Could you check a few things on this model? Use its own coordinates, in mm. A direction names the side the tool comes from. Coordinates: 2 decimals unless noted, no trailing zeros. Order: outer loops, then holes, each group sorted by start corner. A loop starts at its lowest first (then second) coordinate and runs counter-clockwise, first axis right, second up. Notation, with made-up numbers: (44, -19.5) -> (77, -19.5) arc R18 cw to (77, 13.5) -> close; hole circle Ø11 at (46, 6.25). An arc over 180 degrees is marked (long way). Use a Markdown table: item, result. Add a question column.
1) Will these pins go through, and if not, where does the flat tip stop? pin 1 Ø3 at (x, y) = (37, -4.5) entering from +Z; pin 2 Ø4 at (x, y) = (50.8, 0) entering from -Z.
2) If we section it at C-C (y = 0): Give the number of separate pieces and of enclosed holes in the cut face, plus the area to 3 significant figures.
3) Thinking about a two-plate mould opening in Y: for faces 1 (the flat face through (-2, -3, 2.476)), 2 (the cylindrical face through (56.515, -0.087, 0.017)), 3 (the cylindrical face through (23.1, -0.95, 0.62)), which applies, +Y half, -Y half, draft (parallel to the pull), parting line (faces both ways), or undercut?
4) Which directions (+Z, -Z, +X, -X, +Y, -Y) give clear straight access to the entire face, cutting with the end or side of a thin tool? Please do faces 4 (the flat face through (26, 5.588, 0)), 5 (the cylindrical face through (54.57, 0.17, 1.85)).
5) If we section it at A-A (x = 0): Write out the boundary of the cut face in (y, z) (1 decimal), plus the area to 3 significant figures.
6) If we section it at B-B (z = 0): Write out the boundary of the cut face in (x, y).
7) If I drill on L1, parallel to X at y = 0, z = 0.5 (3 decimals); L2, parallel to X at y = 0.5, z = 2.1; L3, parallel to X at y = -1, z = 2.2, over which ranges is the centre line in solid material (lowest first)? Write a range as [from, to].
```python
from build123d import *

# Parameters (mm, degrees)
BOSS_EXTRUDE1_DEPTH = 2.413
SKETCH2_W           = 3.7719
SKETCH2_H           = 1.27
SKETCH3_W           = 3.7719
SKETCH3_H           = 1.27
SKETCH4_W           = 3.7719
SKETCH4_H           = 1.27
HOLE1_D             = 4.97586
HOLE1_CSINK_D       = 6.35
HOLE1_CSINK_ANGLE   = 90
CHAMFER1_SIZE       = 0.68707


with BuildPart() as part:
    # Sketch1 → Boss-Extrude1 (new body)
    with BuildSketch(Plane.XY.offset(1.2065)):
        with BuildLine():
            Line((54.209515887, 5.588), (-3.409515887, 5.588))
            ThreePointArc((-3.409515887, 5.588), (-5.715, 0), (-3.409515887, -5.588))
            Line((-3.409515887, -5.588), (54.209515887, -5.588))
            ThreePointArc((54.209515887, -5.588), (56.515, 0), (54.209515887, 5.588))
        make_face()
    extrude(amount=-BOSS_EXTRUDE1_DEPTH)

    # Sketch2 → Revolve1 (revolve)
    with BuildSketch(Plane.XZ, mode=Mode.PRIVATE) as revolve1_sk:
        with Locations((27.28595, 1.8415)):
            Rectangle(SKETCH2_W, SKETCH2_H)
    revolve(revolve1_sk.sketch.rotate(Axis((25.4, 0, 2.4765), (0, 0, -1)), 180), axis=Axis((25.4, 0, 2.4765), (0, 0, -1)))

    # Sketch3 → Revolve2 (revolve)
    with BuildSketch(Plane.XZ, mode=Mode.PRIVATE) as revolve2_sk:
        with Locations((1.88595, 1.8415)):
            Rectangle(SKETCH3_W, SKETCH3_H)
    revolve(revolve2_sk.sketch.rotate(Axis((0, 0, 2.4765), (0, 0, -1)), 180), axis=Axis((0, 0, 2.4765), (0, 0, -1)))

    # Sketch4 → Revolve3 (revolve)
    with BuildSketch(Plane.XZ, mode=Mode.PRIVATE) as revolve3_sk:
        with Locations((52.68595, 1.8415)):
            Rectangle(SKETCH4_W, SKETCH4_H)
    revolve(revolve3_sk.sketch.rotate(Axis((50.8, 0, 2.4765), (0, 0, -1)), 180), axis=Axis((50.8, 0, 2.4765), (0, 0, -1)))

    # Hole1 (through all)
    with Locations(Plane.XY.offset(2.4765)):
        with Locations((0, 0), (25.4, 0), (50.8, 0)):
            CounterSinkHole(HOLE1_D / 2, HOLE1_CSINK_D / 2, counter_sink_angle=HOLE1_CSINK_ANGLE)

    # Chamfer1
    chamfer1_edges = [part.edges().sort_by_distance(p)[0] for p in [
        (53.28793, 0, -1.2065),
        (27.88793, 0, -1.2065),
        (2.48793, 0, -1.2065),
    ]]
    chamfer(chamfer1_edges, length=CHAMFER1_SIZE)


solid = part.part
```
Answer sheet:
| question | item | result |
|---|---|---|
| 1 | pin 1 | z = 1.21 |
| 1 | pin 2 | through |
| 2 | separate pieces | 4 |
| 2 | enclosed holes | 0 |
| 2 | area | 121 mm2 |
| 3 | face 1 | draft |
| 3 | face 2 | parting line |
| 3 | face 3 | undercut |
| 4 | face 4 | +Z, -Z, +X, -X, +Y |
| 4 | face 5 | +Z |
| 5 | outline | (-5.6, -1.2) -> (-3.2, -1.2) -> (-2.5, -0.5) -> (-2.5, 1.8) -> (-3.2, 2.5) -> (-3.8, 2.5) -> (-3.8, 1.2) -> (-5.6, 1.2) -> close; (2.5, -0.5) -> (3.2, -1.2) -> (5.6, -1.2) -> (5.6, 1.2) -> (3.8, 1.2) -> (3.8, 2.5) -> (3.2, 2.5) -> (2.5, 1.8) -> close |
| 5 | area | 17.3 mm2 |
| 6 | outline | (-3.41, -5.59) -> (54.21, -5.59) arc R7.92 ccw to (54.21, 5.59) -> (-3.41, 5.59) arc R7.92 ccw to start; hole circle Ø4.98 at (0, 0); hole circle Ø4.98 at (25.4, 0); hole circle Ø4.98 at (50.8, 0) |
| 7 | L1 | [-5.715, -2.488], [2.488, 22.912], [27.888, 48.312], [53.288, 56.515] |
| 7 | L2 | [-3.74, -2.75], [2.75, 3.74], [21.66, 22.65], [28.15, 29.14], [47.06, 48.05], [53.55, 54.54] |
| 7 | L3 | [-3.64, -2.72], [2.72, 3.64], [21.76, 22.68], [28.12, 29.04], [47.16, 48.08], [53.52, 54.44] |
